Verification items for the finished model (mm, model axes). Face numbers are marked on the shaded views. A direction names the side the tool comes from. Coordinates: 2 decimals unless noted, no trailing zeros. Write each loop counter-clockwise with the first axis right and the second up, starting at its lowest first coordinate (ties: lowest second). Pieces come first, ordered by that corner, then holes. Notation, with made-up numbers: (42.5, 35) - (82.5, 35) arc R12 cw to (82.5, 53) - close; hole circle Ø8 at (19, 83.25). An arc over 180 degrees is marked (long way). Use one line per item in the form item = value. Start each with the question number.
(1) Material ranges on line 1 (X direction, y = 16.25, z = 0); line 2 (Z direction, x = 0, y = 0.7); line 3 (X direction, y = 9.25, z = -1.5), recorded low to high. Write a range as [from, to].
(2) Mould release check, pull along Z, two halves, no side actions. Record for the marked faces 3, 4, 5 and 6: released by +Z, released by -Z, zero draft, split by the parting line, or undercut.
(3) Tool access check on the marked faces 1 and 2. Record the directions out of +Z, -Z, +X, -X, +Y, -Y that give a thin tool (end or side, any length) a straight path to the whole face; none if there is none.
(4) Sectioned sample at C-C (y = 5). Record the cut outline in (x, z).
(5) Sectioned sample at A-A (x = 0). Count the separate pieces of the cut face and the enclosed holes in it, and give its area (3 significant figures).
from build123d import *

# Parameters (mm, degrees)
SKETCH_1_W               = 12
SKETCH_1_H               = 8
EXTRUDE_1_DEPTH          = 17
CHAMFER_1_SIZE           = 2
SKETCH_3_W               = 8
SKETCH_3_H               = 11
CUT_EXTRUDE_1_DEPTH      = 84.5
CUT_EXTRUDE_2_DEPTH      = 19.466185313
CUT_EXTRUDE_2_DEPTH_BACK = 19.466185313
SKETCH_4_R               = 2
CHAMFER_2_SIZE           = 2


with BuildPart() as part:
    # 草图1 → 凸台-拉伸1 (new body)
    with BuildSketch(Plane(origin=(0, 0, 0), x_dir=(1, 0, 0), z_dir=(0, 1, 0))):
        Rectangle(SKETCH_1_W, SKETCH_1_H)
    extrude(amount=EXTRUDE_1_DEPTH)

    # 倒角1
    chamfer_1_edges = [part.edges().sort_by_distance(p)[0] for p in [
        (6, 8.5, 4),
        (-6, 8.5, 4),
        (-6, 8.5, -4),
        (6, 8.5, -4),
    ]]
    chamfer(chamfer_1_edges, length=CHAMFER_1_SIZE)

    # 草图3 → 切除-拉伸1 (cut, symmetric)
    with BuildSketch(Plane.XY.offset(4)):
        with Locations((0, 8.5)):
            Rectangle(SKETCH_3_W, SKETCH_3_H)
    extrude(amount=CUT_EXTRUDE_1_DEPTH, both=True, mode=Mode.SUBTRACT)

    # 草图4 → 切除-拉伸2 (cut, two sides: drawn at the far end of the back side and taken through both)
    with BuildSketch(Plane(origin=(0, 17, 0), x_dir=(1, 0, 0), z_dir=(0, 1, 0)).offset(-CUT_EXTRUDE_2_DEPTH_BACK)):
        with Locations(Location((0, 0, 0), (0, 0, 270))):
            Circle(SKETCH_4_R)
    extrude(amount=CUT_EXTRUDE_2_DEPTH + CUT_EXTRUDE_2_DEPTH_BACK, mode=Mode.SUBTRACT)

    # 倒角2
    chamfer_2_edges = [part.edges().sort_by_distance(p)[0] for p in [
        (0, 3, -2),
        (0, 14, -2),
    ]]
    chamfer(chamfer_2_edges, length=CHAMFER_2_SIZE - 0.0001)  # a hair under: the kernel refuses the full size


solid = part.part
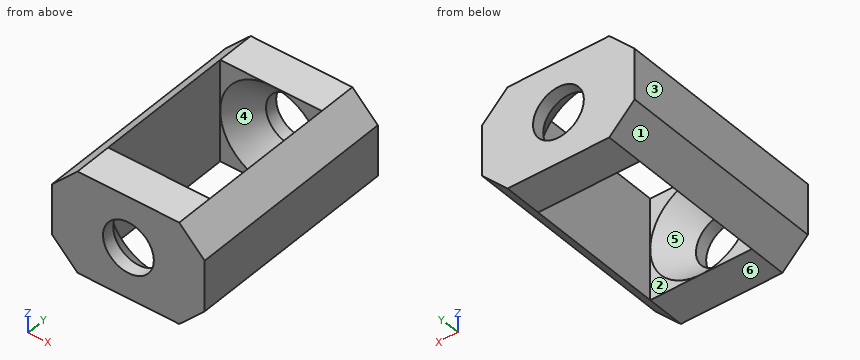
Answers below:
q1.line_1 = [-6, -2], [2, 6]
q1.line_2 = [-4, -2], [2, 4]
q1.line_3 = [-6, -4], [4, 6]
q2.face_3 = zero draft
q2.face_4 = undercut
q2.face_5 = undercut
q2.face_6 = released by -Z
q3.face_1 = -Z, -X, +Y, -Y
q3.face_2 = +Z, -Z
q4.outline = (-6, -2) - (-4, -4) - (-4, 4) - (-6, 2) - close; (4, -4) - (6, -2) - (6, 2) - (4, 4) - close
q5.separate_pieces = 4
q5.enclosed_holes = 0
q5.area = 16.0 mm2
